```python
from build123d import *

# Parameters (mm, degrees)
SKETCH1_W           = 30
SKETCH1_H           = 7.657514459
BOSS_EXTRUDE1_DEPTH = 27.5
FILLET1_R           = 0.5


with BuildPart() as part:
    # Sketch1 → Boss-Extrude1 (new body)
    with BuildSketch(Plane.XY):
        Polygon((-59.54423259, 5.20944533), (-60.873946022, -2.331734278), (-31.329713431, -7.541179608), (-30, 0), align=None)
        Polygon((-30, -7.657514459), (-31.329713431, -7.541179608), (-30, 0), align=None)
        with Locations((-15, -3.82875723)):
            Rectangle(SKETCH1_W, SKETCH1_H)
    extrude(amount=BOSS_EXTRUDE1_DEPTH)

    # Fillet1
    fillet1_edges = [part.edges().sort_by_distance(p)[0] for p in [
        (-60.209089306, 1.438855526, 0),
        (-59.54423259, 5.20944533, 13.75),
        (-30, 0, 13.75),
        (0, 0, 13.75),
        (0, -3.828757229, 27.5),
        (-15, 0, 27.5),
        (-44.772116295, 2.604722665, 27.5),
        (-60.209089306, 1.438855526, 27.5),
        (-44.772116295, 2.604722665, 0),
        (-15, 0, 0),
        (0, -3.828757229, 0),
    ]]
    fillet(fillet1_edges, radius=FILLET1_R)


solid = part.part
```
Geometry check sheet. Reference: the model listing, model coordinates, mm. A direction names the side the tool comes from. Round coordinates to 2 decimals unless told otherwise and drop trailing zeros. Order: outer loops, then holes, each group sorted by start corner. A loop starts at its lowest first (then second) coordinate and runs counter-clockwise, first axis right, second up. Notation, with made-up numbers: (59.5, -37.5) - (81.5, -37.5) arc R20 cw to (81.5, -9.5) - close; hole circle Ø11 at (51, 67). An arc over 180 degrees is marked (long way). Use a Markdown table: item, result. Add a question column.
1) Gauge pin test, flat ends, axial feed: P1, Ø4, axis at y = -3, z = 8.5, coming from the -X side; P2, Ø13, axis at x = -8.5, z = 17, coming from the +Y side. Record the tip position at first contact, or that the pin passes through.
2) Section check C-C (y = -5.25). Record the cut outline in (x, z).
3) Thickness scan on line 1 along Y through (x, z) = (-29, 7.75); line 2 along Y through (x, z) = (-36, 12). Record the ranges inside material, lowest first.
4) Set-up check for faces 1 (the flat face through (-15, 0, 14)), 2 (the flat face through (-30.66, -7.6, 13.56)): record each of +Z, -Z, +X, -X, +Y, -Y from which the full face is reachable in a straight line by a thin tool's end or side.
5) Section check B-B (x = -24.5). Record the cut outline in (y, z).
6) Section check A-A (z = 10.75). Record the cut outline in (x, y).
Established:
| question | item | result |
|---|---|---|
| 1 | P1 | x = -60.87 |
| 1 | P2 | y = 0 |
| 2 | outline | (-44.32, 0) - (-0.5, 0) arc R0.5 ccw to (0, 0.5) - (0, 27) arc R0.5 ccw to (-0.5, 27.5) - (-44.32, 27.5) - close |
| 3 | line 1 | -7.66 to 0 |
| 3 | line 2 | -6.72 to 1.06 |
| 4 | face 1 | +Z, -Z, +X, +Y |
| 4 | face 2 | +Z, -Z, -X, -Y |
| 5 | outline | (-7.66, 0) - (-0.5, 0) arc R0.5 ccw to (0, 0.5) - (0, 27) arc R0.5 ccw to (-0.5, 27.5) - (-7.66, 27.5) - close |
| 6 | outline | (-60.87, -2.33) - (-31.33, -7.54) - (-30, -7.66) - (0, -7.66) - (0, -0.5) arc R0.5 ccw to (-0.5, 0) - (-29.96, 0) arc R0.5 cw to (-30.04, 0.01) - (-59.05, 5.12) arc R0.5 ccw to (-59.63, 4.72) - close |
